Check sheet for the drawn part. Datum: minimum x, y, z corner. Units: mm. Round coordinates to 2 decimals unless told otherwise and drop trailing zeros. Write each loop counter-clockwise with the first axis right and the second up, starting at its lowest first coordinate (ties: lowest second). Pieces come first, ordered by that corner, then holes. Notation, with made-up numbers: M -2.5,42 L 32.5,42 A25 cw 32.5,74 Z; hole C 88,46 d2. An arc over 180 degrees is marked long. One line per item, written item: value. Start each with the question number.
1. Section check C-C (x = 11.5). Record the boundary of the cut face in (y, z) (1 decimal).
2. Section check B-B (x = 21.5). Record the boundary of the cut face in (y, z) (1 decimal).
3. Depth check by flat-ended pin: P1, Ø3, axis at y = 60.5, z = 5.5, coming from the -X side; P2, Ø4, axis at x = 44, z = 6.5, coming from the +Y side; P3, Ø4.5, axis at y = 131, z = 3.5, coming from the +X side; P4, Ø2, axis at x = 24.5, z = 5, coming from the +Y side. Enter the tip coordinate at first touch or a pass-through.
4. Section check A-A (z = 8). Record the boundary of the cut face in (x, y) (1 decimal), and give its area (3 significant figures).
5. Scan lines: probe 1 along Y at (x, z) = (25, 2.75); probe 2 along Y at (x, z) = (19, 6) (1 decimal). Record each from-to range of solid material in increasing order. Write a range as [from, to].
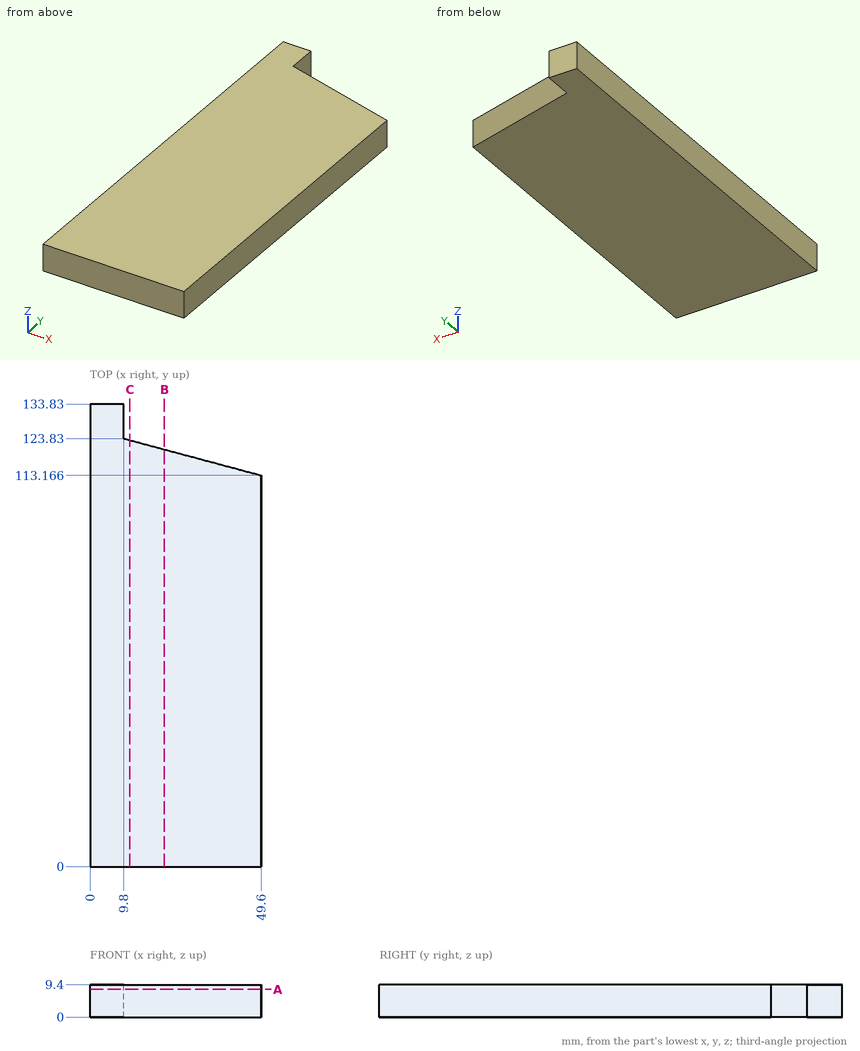
Result sheet:
1. outline: M 0,0 L 123.4,0 L 123.4,9.4 L 0,9.4 Z
2. outline: M 0,0 L 120.7,0 L 120.7,9.4 L 0,9.4 Z
3. P1: stops at x = 0
3. P2: stops at y = 115.2
3. P3: stops at x = 9.8
3. P4: stops at y = 120.16
4. outline: M 0,0 L 49.6,0 L 49.6,113.2 L 9.8,123.8 L 9.8,133.8 L 0,133.8 Z
4. area: 6,030 mm2
5. probe 1: y = [0, 119.76]
5. probe 2: y = [0, 121.4]
